Model file for the job. Use its own axes, mm. A direction names the side the tool comes from. Coordinates: 2 decimals unless noted, no trailing zeros. Put each result on its own line as item: value. Start each with the question number.
1. Drill centre lines: L1, parallel to X at y = 6.5, z = -2.5; L2, parallel to X at y = 12.5, z = 6.25; L3, parallel to Z at x = 17.5, y = 8.5. Where is each one in solid material? Low to high. Write a range as from..to.
2. Pull direction Z, two halves, no side cores. Call faces 4 (the face through (15.24, 6, 0)), 5 (the face through (0, 6, 0)), 6 (the face through (12.95, 2.92, 10.39)), 7 (the face through (17, 6, 3.08)): released by +Z, released by -Z, zero draft, split by the parting line, or undercut.
3. Drop flat-ended pins along their axis: P1, Ø6, axis at x = 5, y = 6.5, coming from the -Z side; P2, Ø10, axis at x = 10, y = 0.5, coming from the +Z side; P3, Ø3, axis at y = 7.5, z = -0.5, coming from the +X side. Give the stop position or say it passes through.
4. Which spindle directions (+Z, -Z, +X, -X, +Y, -Y) get a long thin tool onto all of the face, cutting with end or side? Do faces 1 (the face through (19.05, 9, -2)), 2 (the face through (6.776, 0.053, -0.807)), 3 (the face through (17.17, 3.52, -1.52)). Say none if no direction does.
```python
from build123d import *

# Parameters (mm, degrees)
BOSS_EXTRUDE1_START = 3.81
SKETCH2_R           = 3.81
BOSS_EXTRUDE1_DEPTH = 3.81
FILLET1_R           = 1.016


with BuildPart() as part:
    # Sketch1 → Revolve1 (revolve)
    with BuildSketch(Plane.XY, mode=Mode.PRIVATE) as revolve1_sk:
        with BuildLine():
            Line((0, 0), (0, 6.1976))
            Line((0, 6.1976), (15.24, 6.1976))
            Line((15.24, 6.1976), (15.24, 2.3876))
            Line((15.24, 2.3876), (19.05, 2.3876))
            ThreePointArc((19.05, 2.3876), (17.389827979, -2.102388864), (13.208, -4.4323))
            Line((13.208, -4.4323), (13.208, -4.699))
            Line((13.208, -4.699), (12.7, -4.699))
            Line((12.7, -4.699), (12.7, 0))
            Line((12.7, 0), (0, 0))
        make_face()
    revolve(revolve1_sk.sketch.rotate(Axis((0, 6.1976, 0), (1, 0, 0)), 270), axis=Axis((0, 6.1976, 0), (1, 0, 0)))

    # Sketch2 → Boss-Extrude1 (add)
    with BuildSketch(Plane(origin=(15.24, 0, 0), x_dir=(0, 0, -1), z_dir=(1, 0, 0)).offset(BOSS_EXTRUDE1_START)):
        with Locations((0, 6.1976)):
            Circle(SKETCH2_R)
        Polygon((0, 2.641411017), (3.07975, 4.419505508), (3.07975, 7.975694492), (0, 9.753788983), (-3.07975, 7.975694492), (-3.07975, 4.419505508), align=None, mode=Mode.SUBTRACT)
    extrude(amount=-BOSS_EXTRUDE1_DEPTH)

    # Fillet1
    fillet1_edges = [part.edges().sort_by_distance(p)[0] for p in [
        (0, 6.1976, -6.1976),
    ]]
    fillet(fillet1_edges, radius=FILLET1_R)


solid = part.part
```
Final values:
1. L1: x = 0..15.24
1. L2: x = 12.7..16.84
1. L3: z = -7.84..-2.17, 2.17..7.84
2. face 4: undercut
2. face 5: zero draft
2. face 6: split by the parting line
2. face 7: undercut
3. P1: stops at z = -6.2
3. P2: stops at z = 10.79
3. P3: stops at x = 15.24
4. face 1: +Z, -Z, +X, +Y, -Y
4. face 2: -X
4. face 3: +X
